from build123d import *

# Parameters (mm, degrees)
SKETCH_W        = 25
SKETCH_H        = 18
PAD_DEPTH       = 18
SKETCH001_R     = 2.5
POCKET_DEPTH    = 4
SKETCH002_R     = 3.25
POCKET001_DEPTH = 8.5
SKETCH003_R     = 3.25
POCKET002_DEPTH = 8.5
CHAMFER_SIZE    = 0.4


with BuildPart() as part:
    # Sketch → Pad (new body)
    with BuildSketch(Plane.XY):
        with Locations((22.5, 0)):
            Rectangle(SKETCH_W, SKETCH_H)
    extrude(amount=PAD_DEPTH)

    # Sketch001 (on Face5 of Pad) → Pocket (cut)
    with BuildSketch(Plane(origin=(0, 0, 0), x_dir=(1, 0, 0), z_dir=(0, 0, -1))):
        with Locations((15, 0)):
            Circle(SKETCH001_R)
    extrude(amount=-POCKET_DEPTH, mode=Mode.SUBTRACT)

    # Sketch002 (on Face4 of Pocket) → Pocket001 (cut)
    with BuildSketch(Plane(origin=(0, 0, 0), x_dir=(1, 0, 0), z_dir=(0, 0, -1))):
        with Locations((28, 0)):
            Circle(SKETCH002_R)
    extrude(amount=-POCKET001_DEPTH, mode=Mode.SUBTRACT)

    # Sketch003 (on Face5 of Pocket001) → Pocket002 (cut)
    with BuildSketch(Plane.XY.offset(18)):
        with Locations((20, 0)):
            Circle(SKETCH003_R)
    extrude(amount=-POCKET002_DEPTH, mode=Mode.SUBTRACT)

    # Chamfer
    chamfer_edges = [part.edges().sort_by_distance(p)[0] for p in [
        (22.5, 9, 18),
        (10, 0, 18),
        (35, 0, 18),
        (22.5, -9, 18),
        (16.75, 0, 18),
        (10, -9, 9),
        (10, 9, 9),
        (10, 0, 0),
        (35, -9, 9),
        (22.5, -9, 0),
        (22.5, 9, 0),
        (35, 0, 0),
        (24.75, 0, 0),
        (12.5, 0, 0),
        (35, 9, 9),
    ]]
    chamfer(chamfer_edges, length=CHAMFER_SIZE)


solid = part.part
Could you check a few things on this model? Use its own coordinates, in mm. A direction names the side the tool comes from. Give positions to 0.01 mm unless a question says otherwise; leave off trailing zeros. Loops run counter-clockwise (first coordinate to the right, second up) from the corner with the lowest first, then second, coordinate; pieces in that order, holes last. Notation, with made-up numbers: M 14,-7 L 44,-7 A8 ccw 44,4 Z; hole C 63.5,7 d9. An arc over 180 degrees is marked long. Answer as a JSON object with one key per item and string values.
Q1. If we mould it in two halves opening along Y, with no side actions, what happens to faces 4 (the flat face through (28, 0, 8.5)), 5 (the flat face through (22, 9, 9)), 6 (the cylindrical face through (31.1, -0.98, 4.39)), 7 (the flat face through (25, 0, 18))? For each: pulls with the +Y half, pulls with the -Y half, needs draft (parallel to the pull), parting line crosses it, or undercut.
Values found:
{"face 4": "undercut", "face 5": "pulls with the +Y half", "face 6": "undercut", "face 7": "needs draft"}
Q2. For P1, Ø6, axis at x = 20, y = 0, coming from the +Z side; P2, Ø3, axis at x = 27.5, y = 0, coming from the -Z side, each with a flat end and sliding along its axis, tell me the tip position at first contact or that it passes through.
Values found:
{"P1": "stops at z = 9.5", "P2": "stops at z = 8.5"}
Q3. For faces 1 (the cylindrical face through (12.5, -0.1, 2.2)), 2 (the cylindrical face through (16.753, 0.143, 13.607)), 3 (the flat face through (22, -9, 9)), which set-ups out of +Z, -Z, +X, -X, +Y, -Y let a thin tool reach every point of the face, with its end or its side?
Values found:
{"face 1": "-Z", "face 2": "+Z", "face 3": "+Z, -Z, +X, -X, -Y"}
Q4. If I drill on probe 1 along X at (y, z) = (0, 3.25); probe 2 along Y at (x, z) = (15, 3); probe 3 along Y at (x, z) = (28, 3.75), over which ranges is the centre line in solid material (lowest first)? Write a range as [from, to].
Values found:
{"probe 1": "x = [10, 12.5], [17.5, 24.75], [31.25, 35]", "probe 2": "y = [-9, -2.5], [2.5, 9]", "probe 3": "y = [-9, -3.25], [3.25, 9]"}
Q5. Suppose I cut it at A-A, the plane x = 15. List the corners of the cut face in (y, z) for me.
Values found:
{"outline": "M -9,0.4 L -8.6,0 L -2.9,0 L -2.5,0.4 L -2.5,4 L 2.5,4 L 2.5,0.4 L 2.9,0 L 8.6,0 L 9,0.4 L 9,17.6 L 8.6,18 L -8.6,18 L -9,17.6 Z"}
Q6. Suppose I cut it at C-C, the plane x = 28. List the corners of the cut face in (y, z) for me, plus the area to 3 significant figures.
Values found:
{"outline": "M -9,0.4 L -8.6,0 L -3.65,0 L -3.25,0.4 L -3.25,8.5 L 3.25,8.5 L 3.25,0.4 L 3.65,0 L 8.6,0 L 9,0.4 L 9,17.6 L 8.6,18 L -8.6,18 L -9,17.6 Z", "area": "268 mm²"}
Q7. Suppose I cut it at B-B, the plane z = 11.5. List the corners of the cut face in (x, y) for me.
Values found:
{"outline": "M 10,-8.6 L 10.4,-9 L 34.6,-9 L 35,-8.6 L 35,8.6 L 34.6,9 L 10.4,9 L 10,8.6 Z; hole C 20,0 d6.5"}
